```python
from build123d import *

# Parameters (mm, degrees)
BOSS_EXTRUDE1_DEPTH = 1.5875
SKETCH2_R           = 2.4892
SKETCH2_R_2         = 12.7
CUT_EXTRUDE1_DEPTH  = 4.175
FILLET1_R           = 6.35
CUT_EXTRUDE2_DEPTH  = 4.175
FILLET2_R           = 4.7625


with BuildPart() as part:
    # Sketch1 → Boss-Extrude1 (new body, symmetric)
    with BuildSketch(Plane(origin=(0, 0, 0), x_dir=(1, 0, 0), z_dir=(0, 1, 0))):
        Polygon((0, 0), (0, 203.2), (28.575, 203.2), (28.575, 177.8), (333.375, 177.8), (333.375, 203.2), (371.475, 203.2), (371.475, 152.668916192), (28.575, 0), align=None)
    extrude(amount=BOSS_EXTRUDE1_DEPTH, both=True)

    # Sketch2 → Cut-Extrude1 (cut, through all)
    with BuildSketch(Plane(origin=(0, 1.5875, 0), x_dir=(1, 0, 0), z_dir=(0, 1, 0))):
        with Locations((12.7, 190.5)):
            Circle(SKETCH2_R)
        with Locations((12.7, 165.1)):
            Circle(SKETCH2_R)
        with Locations((12.7, 139.7)):
            Circle(SKETCH2_R)
        with Locations((12.7, 114.3)):
            Circle(SKETCH2_R)
        with Locations((12.7, 88.9)):
            Circle(SKETCH2_R)
        with Locations((12.7, 63.5)):
            Circle(SKETCH2_R)
        with Locations((12.7, 38.1)):
            Circle(SKETCH2_R)
        with Locations((12.7, 12.7)):
            Circle(SKETCH2_R)
        with Locations((352.425, 184.15)):
            Circle(SKETCH2_R_2)
    extrude(amount=-CUT_EXTRUDE1_DEPTH, mode=Mode.SUBTRACT)

    # Fillet1
    fillet1_edges = [part.edges().sort_by_distance(p)[0] for p in [
        (0, 0, 0),
        (0, 0, -203.2),
        (28.575, 0, -203.2),
        (28.575, 0, -177.8),
        (333.375, 0, -177.8),
        (333.375, 0, -203.2),
        (371.475, 0, -203.2),
        (371.475, 0, -152.668916192),
        (28.575, 0, 0),
    ]]
    fillet(fillet1_edges, radius=FILLET1_R)

    # Sketch3 → Cut-Extrude2 (cut, through all)
    with BuildSketch(Plane(origin=(0, 1.5875, 0), x_dir=(1, 0, 0), z_dir=(0, 1, 0))):
        Polygon((29.450902816, 10.816387612), (142.430270713, 61.118043048), (84.86301023, 160.827463057), align=None)
        Polygon((25.4, 18.175792916), (80.844662076, 168.275), (25.4, 168.275), align=None)
        Polygon((144.713091094, 69.864082163), (181.064782686, 168.275), (87.89552119, 168.275), align=None)
        Polygon((149.39765716, 64.220123355), (222.156526072, 96.614458906), (185.08313084, 160.827463057), align=None)
        Polygon((224.439346453, 105.360498021), (247.679131457, 168.275), (188.1156418, 168.275), align=None)
        Polygon((229.123912518, 99.716539213), (275.149004512, 120.208230413), (251.697479611, 160.827463057), align=None)
        Polygon((277.431824893, 128.954269529), (291.956382724, 168.275), (254.729990571, 168.275), align=None)
        Polygon((282.116390959, 123.310310721), (310.372065706, 135.890547641), (295.974730878, 160.827463057), align=None)
        Polygon((312.654886087, 144.636586756), (321.386603328, 168.275), (299.007241838, 168.275), align=None)
        Polygon((325.404951482, 160.827463057), (317.339452153, 138.992627948), (333.784143729, 146.314276359), align=None)
    extrude(amount=-CUT_EXTRUDE2_DEPTH, mode=Mode.SUBTRACT)

    # Fillet2
    fillet2_edges = [part.edges().sort_by_distance(p)[0] for p in [
        (277.431824893, 0, -128.954269529),
        (254.729990571, 0, -168.275),
        (291.956382724, 0, -168.275),
        (229.123912518, 0, -99.716539213),
        (251.697479611, 0, -160.827463057),
        (275.149004512, 0, -120.208230413),
        (312.654886087, 0, -144.636586756),
        (299.007241838, 0, -168.275),
        (321.386603328, 0, -168.275),
        (282.116390959, 0, -123.310310721),
        (295.974730878, 0, -160.827463057),
        (310.372065706, 0, -135.890547641),
        (25.4, 0, -18.175792916),
        (25.4, 0, -168.275),
        (80.844662076, 0, -168.275),
        (144.713091094, 0, -69.864082163),
        (87.89552119, 0, -168.275),
        (181.064782686, 0, -168.275),
        (224.439346453, 0, -105.360498021),
        (188.1156418, 0, -168.275),
        (247.679131457, 0, -168.275),
        (149.39765716, 0, -64.220123355),
        (185.08313084, 0, -160.827463057),
        (222.156526072, 0, -96.614458906),
        (325.404951482, 0, -160.827463057),
        (333.784143729, 0, -146.314276359),
        (317.339452153, 0, -138.992627948),
        (29.450902816, 0, -10.816387612),
        (84.86301023, 0, -160.827463057),
        (142.430270713, 0, -61.118043048),
    ]]
    fillet(fillet2_edges, radius=FILLET2_R)


solid = part.part
```
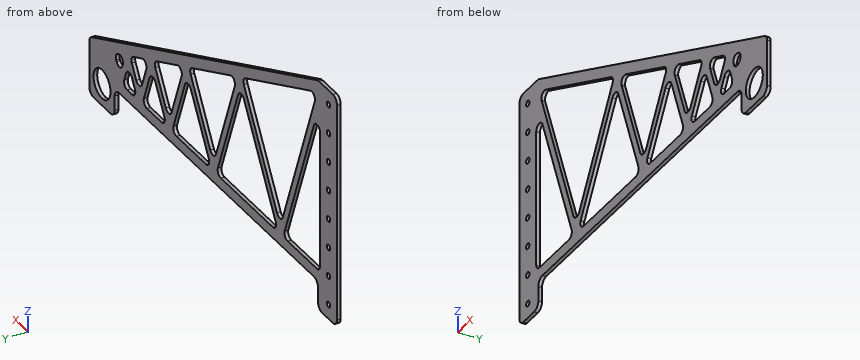
For this review, take the finished solid that the model builds, in its own axes (mm). Round coordinates to 2 decimals unless told otherwise and drop trailing zeros. Use one line per item in the form item = value.
1) Clearance check with flat-ended pins moving along their axes: pin 1 (1.6 mm diameter, centred on x = 276.5, y = 0.5, fed in from +Z); pin 2 (4 mm diameter, centred on x = 12.7, z = -165.1, fed in from +Y) (1 decimal); pin 3 (1.6 mm diameter, centred on x = 311, y = -0.5, fed in from +Z); pin 4 (1.5 mm diameter, centred on x = 213, y = 1, fed in from +Z). State where each tip first meets the part, or that it passes through.
Found:
pin_1 = -110.03
pin_2 = through
pin_3 = -125.39
pin_4 = -81.78
2) To check wall thickness, follow L1, parallel to X at y = 0.45, z = -184.15 (3 decimals); L2, parallel to X at y = 0.3, z = -41; L3, parallel to X at y = 0.9, z = -63.5. State the ranges of each line that lie inside material, in increasing order. Write a range as from..to.
Found:
L1 = 0..28.575, 333.375..339.725, 365.125..371.475
L2 = 0..27.31, 33.02..40.6, 97.24..120.66
L3 = 0..10.21, 15.19..25.4, 42.14..48.91, 140.42..171.2
3) Take a section at A-A, the plane y = 0.1. Count the separate pieces of the cut face and the enclosed holes in it, and give its area (3 significant figures).
Found:
separate_pieces = 1
enclosed_holes = 19
area = 18,100 mm2
